Build history of the part. All positions in model axes, mm. Round coordinates to 2 decimals unless told otherwise and drop trailing zeros. Write each loop counter-clockwise with the first axis right and the second up, starting at its lowest first coordinate (ties: lowest second). Pieces come first, ordered by that corner, then holes. Notation, with made-up numbers: M 17.25,-30 L 47.25,-30 A30 cw 47.25,-1 Z; hole C -29,43 d1. An arc over 180 degrees is marked long. Write item = value, one per line. Start each with the question number.
Q1. Band-saw the part on D-D on z = 2.4. Write the cut outline in (x, y).
Q2. Band-saw the part on C-C on x = 30. Write the cut outline in (y, z).
Q3. Band-saw the part on A-A on x = 9.5. Write the cut outline in (y, z), plus the area to 3 significant figures.
Q4. Drop flat-ended pins along their axis: P1, Ø1.5, axis at x = 8.5, z = 2, coming from the -Y side; P2, Ø0.9, axis at y = 194.5, z = 1.5, coming from the -X side; P3, Ø1.5, axis at y = 203.5, z = 1.5, coming from the +X side. Give the stop position or say it passes through.
Q5. Probe L1, parallel to Y at x = 6, z = 0.2; L2, parallel to X at y = 73.5, z = 2.75; L3, parallel to Y at x = 30, z = 0.65. List the from-to ranges inside material, lowest first.
Q6. Band-saw the part on B-B on y = 117.5. Write the cut outline in (x, z), plus the area to 3 significant figures.
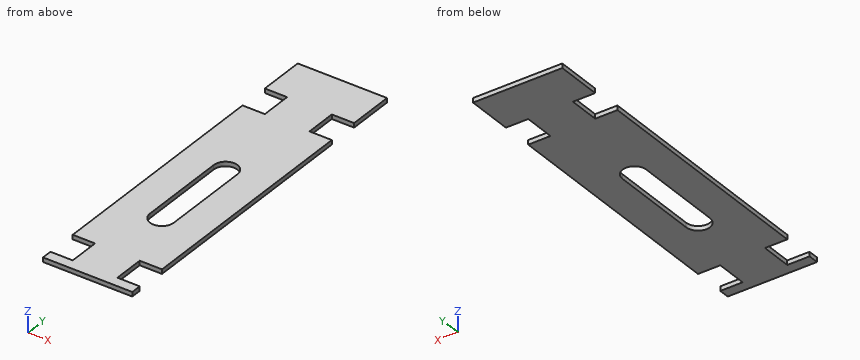
```python
from build123d import *

# Parameters (mm, degrees)
SKETCH_1_W          = 60
SKETCH_1_H          = 240
EXTRUDE_1_DEPTH     = 3
SKETCH_4_W          = 15
SKETCH_4_H          = 21
CUT_EXTRUDE_1_DEPTH = 3


with BuildPart() as part:
    # 草图1 → 凸台-拉伸1 (new body)
    with BuildSketch(Plane.XY):
        with Locations((30, 120)):
            Rectangle(SKETCH_1_W, SKETCH_1_H)
    extrude(amount=EXTRUDE_1_DEPTH)

    # 草图4 → 切除-拉伸1 (cut)
    with BuildSketch(Plane(origin=(0, 0, 0), x_dir=(-1, 0, 0), z_dir=(0, 0, -1))):
        with Locations((-52.5, 17.5)):
            Rectangle(SKETCH_4_W, SKETCH_4_H)
        with Locations((-7.5, 17.5)):
            Rectangle(SKETCH_4_W, SKETCH_4_H)
        with Locations((-7.5, 198.5)):
            Rectangle(SKETCH_4_W, SKETCH_4_H)
        with Locations((-52.5, 198.5)):
            Rectangle(SKETCH_4_W, SKETCH_4_H)
        with BuildLine():
            Line((-22, 130), (-22, 70))
            ThreePointArc((-22, 70), (-30, 62), (-38, 70))
            Line((-38, 70), (-38, 130))
            ThreePointArc((-38, 130), (-30, 138), (-22, 130))
        make_face()
    extrude(amount=-CUT_EXTRUDE_1_DEPTH, mode=Mode.SUBTRACT)


solid = part.part
```
Conclusion:
q1.outline = M 0,0 L 60,0 L 60,7 L 45,7 L 45,28 L 60,28 L 60,188 L 45,188 L 45,209 L 60,209 L 60,240 L 0,240 L 0,209 L 15,209 L 15,188 L 0,188 L 0,28 L 15,28 L 15,7 L 0,7 Z; hole M 22,70 A8 ccw 38,70 L 38,130 A8 ccw 22,130 Z
q2.outline = M 0,0 L 62,0 L 62,3 L 0,3 Z; M 138,0 L 240,0 L 240,3 L 138,3 Z
q3.outline = M 0,0 L 7,0 L 7,3 L 0,3 Z; M 28,0 L 188,0 L 188,3 L 28,3 Z; M 209,0 L 240,0 L 240,3 L 209,3 Z
q3.area = 594 mm^2
q4.P1 = 0
q4.P2 = 15
q4.P3 = 45
q5.L1 = 0 to 7, 28 to 188, 209 to 240
q5.L2 = 0 to 22, 38 to 60
q5.L3 = 0 to 62, 138 to 240
q6.outline = M 0,0 L 22,0 L 22,3 L 0,3 Z; M 38,0 L 60,0 L 60,3 L 38,3 Z
q6.area = 132 mm^2
